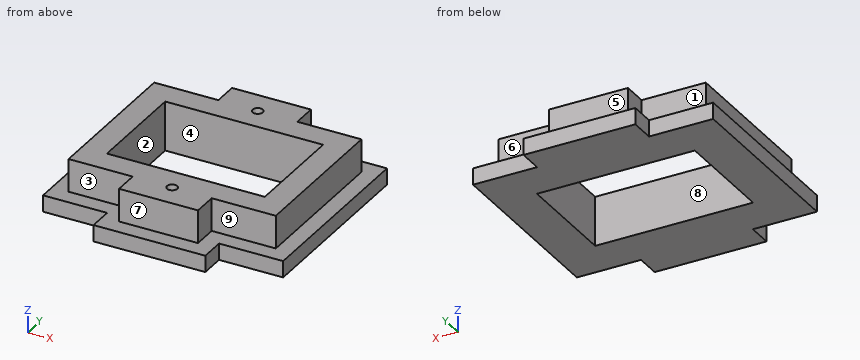
```python
from build123d import *

# Parameters (mm, degrees)
SKETCH1_R           = 0.5
SKETCH1_W           = 15.24
SKETCH1_H           = 10.16
BOSS_EXTRUDE1_DEPTH = 3.175
SKETCH2_W           = 15.24
SKETCH2_H           = 10.16
BOSS_EXTRUDE2_DEPTH = 1.5875


with BuildPart() as part:
    # Sketch1 → Boss-Extrude1 (new body)
    with BuildSketch(Plane.XY):
        Polygon((3.81, -7.46125), (10.00125, -7.46125), (10.00125, 7.46125), (3.81, 7.46125), (3.81, 9.8425), (-3.81, 9.8425), (-3.81, 7.46125), (-10.00125, 7.46125), (-10.00125, -7.46125), (-3.81, -7.46125), (-3.81, -9.8425), (3.81, -9.8425), align=None)
        with Locations((0, 7.46125)):
            Circle(SKETCH1_R, mode=Mode.SUBTRACT)
        with Locations((0, -7.46125)):
            Circle(SKETCH1_R, mode=Mode.SUBTRACT)
        Rectangle(SKETCH1_W, SKETCH1_H, mode=Mode.SUBTRACT)
    extrude(amount=BOSS_EXTRUDE1_DEPTH)

    # Sketch2 → Boss-Extrude2 (add)
    with BuildSketch(Plane(origin=(0, 0, 0), x_dir=(-1, 0, 0), z_dir=(0, 0, -1))):
        Polygon((5.3975, -9.04875), (11.58875, -9.04875), (11.58875, 9.04875), (5.3975, 9.04875), (5.3975, 11.43), (-5.3975, 11.43), (-5.3975, 9.04875), (-11.58875, 9.04875), (-11.58875, -9.04875), (-5.3975, -9.04875), (-5.3975, -11.43), (5.3975, -11.43), align=None)
        Rectangle(SKETCH2_W, SKETCH2_H, mode=Mode.SUBTRACT)
    extrude(amount=BOSS_EXTRUDE2_DEPTH)


solid = part.part
```
Geometry check sheet. Reference: the model listing, model coordinates, mm. Face numbers are marked on the shaded views. A direction names the side the tool comes from. Coordinates: 2 decimals unless noted, no trailing zeros. Write each loop counter-clockwise with the first axis right and the second up, starting at its lowest first coordinate (ties: lowest second). Pieces come first, ordered by that corner, then holes. Notation, with made-up numbers: (34.5, 29) -> (55.5, 29) arc R10 ccw to (55.5, 42) -> close; hole circle Ø4 at (46, 84). An arc over 180 degrees is marked (long way). Use CSV: the item, a comma, the result in double quotes. Start each with the question number.
Item 1: Cross-section at C-C, the plane y = 3.5. Record the cut outline in (x, z) (1 decimal).
Item 2: Cross-section at B-B, the plane z = 0.3. Record the cut outline in (x, y).
Item 3: Set-up check for the marked faces 5, 6, 7, 8 and 9: record each of +Z, -Z, +X, -X, +Y, -Y from which the full face is reachable in a straight line by a thin tool's end or side.
Item 4: Cross-section at A-A, the plane x = 1.5. Record the cut outline in (y, z) (1 decimal), plus the area to 3 significant figures.
Item 5: Depth check by flat-ended pin: pin 1 Ø1.5 at (y, z) = (-2, 1.5) entering from +X; pin 2 Ø0.5 at (y, z) = (10, -1) entering from +X; pin 3 Ø1.7 at (x, z) = (-8.5, -0.5) entering from +Y. Enter the tip coordinate at first touch or a pass-through.
Item 6: Thickness scan on line 1 (Y direction, x = 0, z = 1.1); line 2 (X direction, y = 1, z = 0.65); line 3 (Y direction, x = 3.25, z = -0.5). Record the ranges inside material, lowest first.
Item 7: Cross-section at D-D, the plane y = 6.25. Record the cut outline in (x, z) (1 decimal), plus the area to 3 significant figures.
Item 8: Mould release check, pull along Y, two halves, no side actions. Record for the marked faces 1, 2, 3 and 4: released by +Y, released by -Y, zero draft, split by the parting line, or undercut.
Answers:
1,outline,"(-11.6, -1.6) -> (-7.6, -1.6) -> (-7.6, 3.2) -> (-10, 3.2) -> (-10, 0) -> (-11.6, 0) -> close; (7.6, -1.6) -> (11.6, -1.6) -> (11.6, 0) -> (10, 0) -> (10, 3.2) -> (7.6, 3.2) -> close"
2,outline,"(-10, -7.46) -> (-3.81, -7.46) -> (-3.81, -9.84) -> (3.81, -9.84) -> (3.81, -7.46) -> (10, -7.46) -> (10, 7.46) -> (3.81, 7.46) -> (3.81, 9.84) -> (-3.81, 9.84) -> (-3.81, 7.46) -> (-10, 7.46) -> close; hole (-7.62, -5.08) -> (7.62, -5.08) -> (7.62, 5.08) -> (-7.62, 5.08) -> close; hole circle Ø1 at (0, -7.46); hole circle Ø1 at (0, 7.46)"
3,face 5,"+Z, +X, -X, +Y"
3,face 6,"+Z, +X, +Y"
3,face 7,"+Z, +X, -X, -Y"
3,face 8,"+Z, -Z"
3,face 9,"+Z, +X, -Y"
4,outline,"(-11.4, -1.6) -> (-5.1, -1.6) -> (-5.1, 3.2) -> (-9.8, 3.2) -> (-9.8, 0) -> (-11.4, 0) -> close; (5.1, -1.6) -> (11.4, -1.6) -> (11.4, 0) -> (9.8, 0) -> (9.8, 3.2) -> (5.1, 3.2) -> close"
4,area,"50.4 mm^2"
5,pin 1,"x = 10"
5,pin 2,"x = 5.4"
5,pin 3,"y = 9.05"
6,line 1,"-9.84 to -7.96, -6.96 to -5.08, 5.08 to 6.96, 7.96 to 9.84"
6,line 2,"-10 to -7.62, 7.62 to 10"
6,line 3,"-11.43 to -5.08, 5.08 to 11.43"
7,outline,"(-11.6, -1.6) -> (11.6, -1.6) -> (11.6, 0) -> (10, 0) -> (10, 3.2) -> (-10, 3.2) -> (-10, 0) -> (-11.6, 0) -> close"
7,area,"100 mm^2"
8,face 1,"released by +Y"
8,face 2,"undercut"
8,face 3,"released by -Y"
8,face 4,"undercut"
